Here's how the part is built. I have some questions about the finished solid (model axes, mm). Coordinates: 2 decimals unless noted, no trailing zeros. Write each question's results on one line, items separated by ' | '. Start each with the question number.
from build123d import *

# Parameters (mm, degrees)
F0_W     = 304.8
F0_H     = 101.6
F1_DEPTH = 6.35
F2_R     = 3.175
F3_DEPTH = 6.35
F4_R     = 14.2875
F5_DEPTH = 6.35
F6_R     = 3.0861
F7_DEPTH = 6.35


with BuildPart() as f1:
    # F0 (on Top) → F1 (new body)
    with BuildSketch(Plane.XY):
        with Locations((79.710026, -8.171286)):
            Rectangle(F0_W, F0_H)
    extrude(amount=F1_DEPTH)

    # F2 (on face) → F3 (cut)
    with BuildSketch(Plane.XY.offset(6.35)):
        with Locations((-47.289974, -8.171286)):
            Circle(F2_R)
    extrude(amount=-F3_DEPTH, mode=Mode.SUBTRACT)

    # F4 (on face) → F5 (cut)
    with BuildSketch(Plane.XY.offset(6.35)):
        with Locations((194.010026, -8.171286)):
            Circle(F4_R)
    extrude(amount=-F5_DEPTH, mode=Mode.SUBTRACT)

    # F6 (on face) → F7 (cut)
    with BuildSketch(Plane.XY.offset(6.35)):
        with Locations((105.110026, -8.171286)):
            Circle(F6_R)
    extrude(amount=-F7_DEPTH, mode=Mode.SUBTRACT)


solid = f1.part
1) I want a section at A-A, the plane z = 2.5. Give the number of separate pieces and of enclosed holes in the cut face, then the cut area to 3 significant figures.
2) Please list where this line runs through material, in increasing order: line 1 (Y direction, x = 184, z = 5.5). Write a range as [from, to].
3) We'd pull the mould along Y, two halves only. Please class faces 1 (the flat face through (232.11, -9, 3)), 2 (the flat face through (78, 42.629, 3)), 3 (the cylindrical face through (179.736, -7.543, 3.219)): pulls with the +Y half, pulls with the -Y half, needs draft (parallel to the pull), parting line crosses it, or undercut.
Output:
1) separate pieces: 1 | enclosed holes: 3 | area: 30,300 mm2
2) line 1: y = [-58.97, -18.37], [2.02, 42.63]
3) face 1: needs draft | face 2: pulls with the +Y half | face 3: undercut
